Autodesk Inventor part; units mm, degrees
ref_plane "Počáteční rovina" through (0, 0, 0) normal (0, 0, 1) x (1, 0, 0)
ref_plane "Koncová rovina" through (0, 0, 875) normal (0, 0, 1) x (1, 0, 0)
ref_plane "Pracovní rovina4" through (417.5, -11.5, 435) normal (0, 0, 1) x (0, -1, 0)
ref_plane "Počáteční rovina" through (0, 0, 0) normal (0, 0, 1) x (1, 0, 0)
ref_plane "Koncová rovina" through (0, 0, 875) normal (0, 0, 1) x (1, 0, 0)
sketch "Náčrt1" plane through (0, 0, 0) normal (0, 0, 1) x (1, 0, 0)
  line L0 (-11.5, 17.5) -> (11.5, 17.5)
  line L1 (17.5, 11.5) -> (17.5, -11.5)
  line L2 (11.5, -17.5) -> (-11.5, -17.5)
  line L3 (-17.5, -11.5) -> (-17.5, 11.5)
  arc A0 (-11.5, 17.5) -> (-17.5, 11.5) centre (-11.5, 11.5) ccw
  arc A1 (17.5, 11.5) -> (11.5, 17.5) centre (11.5, 11.5) ccw
  arc A2 (11.5, -17.5) -> (17.5, -11.5) centre (11.5, -11.5) ccw
  arc A3 (-17.5, -11.5) -> (-11.5, -17.5) centre (-11.5, -11.5) ccw
  line L4 (-26.2397, 0) -> (26.2397, 0) construction
  line L5 (0, -26.2397) -> (0, 26.2397) construction
  arc A4 (-11.5, 14.5) -> (-14.5, 11.5) centre (-11.5, 11.5) ccw
  line L6 (-11.5, 14.5) -> (11.5, 14.5)
  arc A5 (14.5, 11.5) -> (11.5, 14.5) centre (11.5, 11.5) ccw
  line L7 (14.5, 11.5) -> (14.5, -11.5)
  arc A6 (11.5, -14.5) -> (14.5, -11.5) centre (11.5, -11.5) ccw
  line L8 (11.5, -14.5) -> (-11.5, -14.5)
  arc A7 (-14.5, -11.5) -> (-11.5, -14.5) centre (-11.5, -11.5) ccw
  line L9 (-14.5, -11.5) -> (-14.5, 11.5)
  point P0 (-17.5, 17.5)
  point P1 (17.5, -17.5)
  point P2 (17.5, 17.5)
  dimension "b" = 35
  dimension "msp_r" = 6
  dimension "d8" = 17.5
  dimension "d9" = 17.5
  dimension "d10" = 3
extrude "Těleso" add sketch "Náčrt1" along normal blind 870
sketch "Sketch2" plane through (0, 0, 0) normal (0, 0, 1) x (1, 0, 0)
  line L0 (0, 0) -> (10, 0)
ref_plane "Work Plane3" through (0, 0, 0) normal (0, -1, 0) x (1, 0, 0)
sketch "Sketch3" plane through (0, 0, 0) normal (0, -1, 0) x (1, 0, 0)
  line L0 (-2, 0) -> (12, 0)
  line L1 (-2, 875) -> (12, 875)
  dimension "d14" = 875
sketch "Náčrt4" plane through (11.5, 17.5, 875) normal (0, 1, 0) x (1, 0, 0)
  line L0 (-29, 875) -> (-29, 5) construction
  line L1 (6, 875) -> (6, 5) construction
  line L2 (-29, 875) -> (6, 875)
  line L3 (6, 875) -> (6, 840)
  line L4 (-29, 875) -> (-29, 5) construction
  line L5 (6, 840) -> (-29, 875)
  line L6 (6, 875) -> (6, 5) construction
  line L7 (-23, 5) -> (-29, 5)
  line L8 (-29, 5) -> (6, 40)
  line L9 (6, 40) -> (6, 5)
  line L10 (6, 5) -> (-29, 5)
  point P0 (-11.5, 875)
  dimension "d15" = 45
  dimension "d19" = 45
extrude "Vysunutí2" cut sketch "Náčrt4" against normal through all
ref_plane "Pracovní rovina4" through (417.5, -11.5, 435) normal (0, 0, 1) x (0, -1, 0)
equation "\"msp_r\" = 2 * ParT"
equation "\"d8\" = d9"
equation "\"d9\" = 0.5 * b"
equation "\"d10\" = ParT"
equation "\"G_OFFSET_START\" = 0"
equation "\"G_OFFSET_END\" = 0"
equation "\"d12\" = G_OFFSET_END + B_L"
equation "\"G_L\" = d14"
equation "\"B_L\" = 875"
equation "\"PoloměrOhybu\" = Tloušťka"
equation "\"ŠířkaVýštipu\" = Tloušťka"
equation "\"HloubkaVýštipu\" = 0.5 * Tloušťka"
equation "\"VelikostRohovéhoVýštipu\" = 4 * Tloušťka"
equation "\"MinimálníZbytek\" = 2 * Tloušťka"
equation "\"PřechodovýPoloměr\" = PoloměrOhybu"
equation "\"VelikostJacobihoPoloměru\" = Tloušťka"
equation "\"VelikostMezery\" = Tloušťka"
properties part number "DD_KVD_003_02" material "Nerezová ocel"
Read the model definition and answer for the solid it produces. Units are mm, in the model's axes. A direction names the side the tool comes from. Give positions to 0.01 mm unless a question says otherwise; leave off trailing zeros. Write each loop counter-clockwise with the first axis right and the second up, starting at its lowest first coordinate (ties: lowest second). Pieces come first, ordered by that corner, then holes. Notation, with made-up numbers: (-25.5, 13) - (-17.5, 13) arc R18 cw to (-17.5, 18) - close; hole circle Ø10 at (-28.5, -15.75). An arc over 180 degrees is marked (long way). Return JSON: item names as keys, results as strings.
Q1. Consider line 1 along Y through (x, z) = (10, 714); line 2 along Y through (x, z) = (13.5, 574.5). Determine where each line is inside the solid, lowest interval first. Write a range as [from, to].
Reply:
{"line 1": "[-17.5, -14.5], [14.5, 17.5]", "line 2": "[-17.16, -13.74], [13.74, 17.16]"}
Q2. For a pull along Y with two mould halves and no side action, classify faces 3 (the face through (0, -17.5, 429)), 4 (the face through (0, 14.5, 429)), 5 (the face through (-17.5, 0, 429)) as released by +Y, released by -Y, zero draft, split by the parting line, or undercut.
Reply:
{"face 3": "released by -Y", "face 4": "undercut", "face 5": "zero draft"}
Q3. Given P1, Ø10, axis at x = 5, y = 11, coming from the -Z side, flat-ended and moving along its own axis, determine where the tip first touches the part or whether it passes through.
Reply:
{"P1": "z = 18.93"}
Q4. A cutting plane is placed at A-A, the plane y = 2. Determine the outline of the cut face in (x, z), and give its area (3 significant figures).
Reply:
{"outline": "(-17.5, 0) - (-14.5, 3) - (-14.5, 867) - (-17.5, 870) - close; (14.5, 32) - (17.5, 35) - (17.5, 835) - (14.5, 838) - close", "area": "5,010 mm²"}
Q5. A cutting plane is placed at B-B, the plane x = -4.5. Determine the outline of the cut face in (y, z), and give its area (3 significant figures).
Reply:
{"outline": "(-17.5, 13) - (-14.5, 13) - (-14.5, 857) - (-17.5, 857) - close; (14.5, 13) - (17.5, 13) - (17.5, 857) - (14.5, 857) - close", "area": "5,060 mm²"}
Q6. For faces 1 (the face through (17.5, 0, 429)), 2 (the face through (0, -14.5, 429)), determine the directions among +Z, -Z, +X, -X, +Y, -Y from which every point of the face is accessible in a straight line to the end or side of a thin tool.
Reply:
{"face 1": "+Z, -Z, +X, +Y, -Y", "face 2": "+Z, -Z"}
Q7. A cutting plane is placed at C-C, the plane z = 661. Determine the outline of the cut face in (x, y), and give its area (3 significant figures).
Reply:
{"outline": "(-17.5, -11.5) arc R6 ccw to (-11.5, -17.5) - (11.5, -17.5) arc R6 ccw to (17.5, -11.5) - (17.5, 11.5) arc R6 ccw to (11.5, 17.5) - (-11.5, 17.5) arc R6 ccw to (-17.5, 11.5) - close; hole (-14.5, -11.5) arc R3 ccw to (-11.5, -14.5) - (11.5, -14.5) arc R3 ccw to (14.5, -11.5) - (14.5, 11.5) arc R3 ccw to (11.5, 14.5) - (-11.5, 14.5) arc R3 ccw to (-14.5, 11.5) - close", "area": "361 mm²"}
